Could you check a few things on this model? Use its own coordinates, in mm. A direction names the side the tool comes from. Round coordinates to 2 decimals unless told otherwise and drop trailing zeros. Loops run counter-clockwise (first coordinate to the right, second up) from the corner with the lowest first, then second, coordinate; pieces in that order, holes last. Notation, with made-up numbers: (-24, 80.25) -> (34, 80.25) arc R15 cw to (34, 92.25) -> close; hole circle Ø8 at (-34, 18). An arc over 180 degrees is marked (long way). One line per item, written item: value.
```python
from build123d import *

# Parameters (mm, degrees)
F0_W      = 698.5
F0_H      = 406.4
F1_DEPTH  = 25.4
F3_DEPTH  = 25.4
F4_W      = 12.7
F4_H      = 254
F5_DEPTH  = 25.4
F6_R      = 50.8
F7_W      = 76.2
F7_H      = 127
F8_DEPTH  = 25.4
F9_R      = 25.4
F10_R     = 25.4
F12_DEPTH = 25.401


with BuildPart() as f1:
    # F0 (on Top) → F1 (new body)
    with BuildSketch(Plane.XY):
        with Locations((62.9796185677, -1.3083405793)):
            Rectangle(F0_W, F0_H)
    extrude(amount=F1_DEPTH)

    # F2 (on face) → F3 (cut)
    with BuildSketch(Plane.XY.offset(25.4)):
        with BuildLine():
            Line((336.0296185677, 284.5435195792), (336.0296185677, 77.4316594207))
            ThreePointArc((336.0296185677, 77.4316594207), (338.3263876052, 70.1472386791), (344.3859627474, 65.4975631367))
            Line((344.3859627474, 65.4975631367), (488.1807398124, 13.1605444421))
            Line((488.1807398124, 13.1605444421), (504.1641078178, 284.5435195792))
            Line((504.1641078178, 284.5435195792), (336.0296185677, 284.5435195792))
        make_face()
    extrude(amount=-F3_DEPTH, mode=Mode.SUBTRACT)

    # F4 (on face) → F5 (cut)
    with BuildSketch(Plane.XY.offset(25.4)):
        with Locations((405.8796185677, -77.5083405793)):
            Rectangle(F4_W, F4_H)
    extrude(amount=-F5_DEPTH, mode=Mode.SUBTRACT)

    # F6
    f6_edges = [f1.edges().sort_by_distance(p)[0] for p in [
        (336.029619, 201.891659, 12.7),
    ]]
    fillet(f6_edges, radius=F6_R)

    # F7 (on face) → F8 (cut)
    with BuildSketch(Plane.XY.offset(25.4)):
        with Locations((-248.1703814323, 138.3916594207)):
            Rectangle(F7_W, F7_H)
    extrude(amount=-F8_DEPTH, mode=Mode.SUBTRACT)

    # F9
    f9_edges = [f1.edges().sort_by_distance(p)[0] for p in [
        (-210.070381, 74.891659, 12.7),
    ]]
    fillet(f9_edges, radius=F9_R)

    # F10
    f10_edges = [f1.edges().sort_by_distance(p)[0] for p in [
        (-210.070381, 201.891659, 12.7),
        (-286.270381, 74.891659, 12.7),
        (399.529619, 45.426914, 12.7),
    ]]
    fillet(f10_edges, radius=F10_R)

    # F11 (on face) → F12 (cut, through all)
    with BuildSketch(Plane.XY.offset(25.4)):
        with BuildLine():
            Line((62.9796185677, -212.4609104405), (62.9796185677, -153.7083405793))
            ThreePointArc((62.9796185677, -153.7083405793), (56.6296185677, -147.3583405793), (50.2796185677, -153.7083405793))
            Line((50.2796185677, -153.7083405793), (50.2796185677, -204.7673902215))
            Line((50.2796185677, -204.7673902215), (62.9796185677, -212.4609104405))
        make_face()
    extrude(amount=-F12_DEPTH, mode=Mode.SUBTRACT)


solid = f1.part
```
Item 1: I need wall thicknesses on line 1 (Y direction, x = -236, z = 7.75); line 2 (X direction, y = -161, z = 10.5); line 3 (X direction, y = 103.5, z = 22). Which ranges of each line are inside material? Lowest first, please. Write a range as from..to.
Output:
line 1: y = -204.51..74.89
line 2: x = -286.27..50.28, 62.98..399.53
line 3: x = -210.07..336.03
Item 2: Will these pins go through, and if not, where does the flat tip stop? pin 1 Ø4 at (y, z) = (145.5, 16) entering from +X; pin 2 Ø7.5 at (x, z) = (-249.5, 14) entering from +Y.
Output:
pin 1: stops at x = 336.03
pin 2: stops at y = 74.89
Item 3: If we mould it in two halves opening along X, with no side actions, what happens to faces 1 (the face through (320.75, 187.41, 12.88)), 2 (the face through (-202.83, 194.25, 12.52)), 3 (the face through (50.28, -179, 13)), 4 (the face through (52, 2, 0))? For each: released by +X, released by -X, zero draft, split by the parting line, or undercut.
Output:
face 1: released by +X
face 2: released by -X
face 3: undercut
face 4: zero draft
Item 4: For faces 5 (the face through (399.53, -90, 13)), 6 (the face through (-210.07, 138, 13)), 7 (the face through (-286.27, -79, 13)), 8 (the face through (336.03, 115, 13)), 9 (the face through (62.98, -179, 13)), which set-ups out of +Z, -Z, +X, -X, +Y, -Y let a thin tool reach every point of the face, with its end or its side?
Output:
face 5: +Z, -Z, +X, +Y, -Y
face 6: +Z, -Z, -X, +Y
face 7: +Z, -Z, -X, +Y, -Y
face 8: +Z, -Z, +X, +Y
face 9: +Z, -Z, -Y
Item 5: If we section it at B-B on y = -163: List the corners of the cut face in (x, z) for me, plus the area to 3 significant figures.
Output:
outline: (-286.27, 0) -> (50.28, 0) -> (50.28, 25.4) -> (-286.27, 25.4) -> close; (62.98, 0) -> (399.53, 0) -> (399.53, 25.4) -> (62.98, 25.4) -> close
area: 17,100 mm²
Item 6: If we section it at D-D on x = -218: List the corners of the cut face in (y, z) for me, plus the area to 3 significant figures.
Output:
outline: (-204.51, 0) -> (81.85, 0) -> (81.85, 25.4) -> (-204.51, 25.4) -> close
area: 7,270 mm²
Item 7: If we section it at A-A on z = 12: List the corners of the cut face in (x, y) for me.
Output:
outline: (-286.27, -204.51) -> (50.28, -204.51) -> (50.28, -153.71) arc R6.35 cw to (62.98, -153.71) -> (62.98, -204.51) -> (399.53, -204.51) -> (399.53, 27.64) arc R25.4 ccw to (382.82, 51.51) -> (344.39, 65.5) arc R12.7 cw to (336.03, 77.43) -> (336.03, 151.09) arc R50.8 ccw to (285.23, 201.89) -> (-184.67, 201.89) arc R25.4 ccw to (-210.07, 176.49) -> (-210.07, 100.29) arc R25.4 cw to (-235.47, 74.89) -> (-260.87, 74.89) arc R25.4 ccw to (-286.27, 49.49) -> close
Item 8: If we section it at C-C on y = 124: List the corners of the cut face in (x, z) for me.
Output:
outline: (-210.07, 0) -> (336.03, 0) -> (336.03, 25.4) -> (-210.07, 25.4) -> close
